Build history of the part. All positions in model axes, mm. Face numbers are marked on the shaded views. A direction names the side the tool comes from. Round coordinates to 2 decimals unless told otherwise and drop trailing zeros. Write each loop counter-clockwise with the first axis right and the second up, starting at its lowest first coordinate (ties: lowest second). Pieces come first, ordered by that corner, then holes. Notation, with made-up numbers: (10, -10) - (52, -10) arc R17 cw to (52, 6) - close; hole circle Ø2 at (-8.75, 44.5). An arc over 180 degrees is marked (long way). Answer as a JSON object with one key per item and string values. Group by question number.
Item 1: Slice it at C-C, the plane y = -14.5. List the corners of the cut face in (x, z), then the cut area to 3 significant figures.
Item 2: Slice it at A-A, the plane y = -4.5. List the corners of the cut face in (x, z).
Item 3: Which spindle directions (+Z, -Z, +X, -X, +Y, -Y) get a long thin tool onto all of the face, cutting with end or side? Do the marked faces 4 and 5. Say none if no direction does.
Item 4: Two-plate mould, pull along Z, no slides. Class the marked faces 1, 2 and 3: +Z half, -Z half, draft (parallel to the pull), parting line (faces both ways), or undercut.
Item 5: Slice it at B-B, the plane y = -10. List the corners of the cut face in (x, z), then the cut area to 3 significant figures.
Item 6: Flat gauge pins, fed straight in: pin 1 (6 mm diameter, centred on x = 13.5, y = -12, fed in from -Z); pin 2 (8 mm diameter, centred on x = 15, y = -11, fed in from -Z); pin 3 (4 mm diameter, centred on x = -0.5, y = -5.5, fed in from -Z). Where does each tip first touch, or does it go through?
Item 7: Probe line 1 (X direction, y = -11.5, z = 0); line 2 (X direction, y = -11.25, z = -2); line 3 (Z direction, x = 2.5, y = -7.75). List the from-to ranges inside material, lowest first. Write a range as from..to.
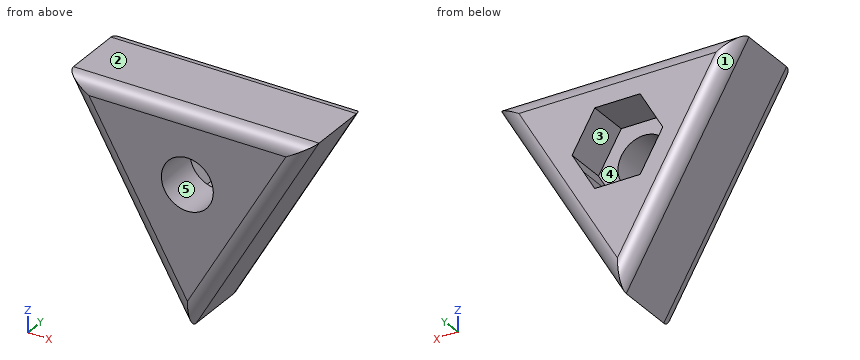
from build123d import *

# Parameters (mm, degrees)
F2_DEPTH = 15.875
F3_DEPTH = 7.62
F4_R     = 4.699
F5_DEPTH = 25.4
F6_R     = 2.54


with BuildPart() as f2:
    # F0 (on Front) → F2 (new body)
    with BuildSketch(Plane.XZ):
        Polygon((22.232984, 12.827), (-22.217016, 12.827), (0.007984, -25.667829), align=None)
    extrude(amount=F2_DEPTH)

    # F1 (on Front) → F3 (cut)
    with BuildSketch(Plane.XZ):
        Polygon((6.159173, -3.556), (8.21223, 0), (4.106115, 7.112), (-4.106115, 7.112), (-8.21223, 0), (-4.106115, -7.112), (4.106115, -7.112), align=None)
    extrude(amount=F3_DEPTH, mode=Mode.SUBTRACT)

    # F4 (on Front) → F5 (cut)
    with BuildSketch(Plane.XZ):
        Circle(F4_R)
    extrude(amount=F5_DEPTH, mode=Mode.SUBTRACT)

    # F6
    f6_edges = [f2.edges().sort_by_distance(p)[0] for p in [
        (-11.104516, 0, -6.420415),
        (0.007984, 0, 12.827),
        (11.120484, 0, -6.420415),
        (0.007984, -15.875, 12.827),
        (-11.104516, -15.875, -6.420415),
        (11.120484, -15.875, -6.420415),
    ]]
    fillet(f6_edges, radius=F6_R)


solid = f2.part
Geometry says:
{
 "1": {"outline": "(-21.73, 12.54) - (0.01, -25.1) - (21.74, 12.54) - close; hole circle Ø9.4 at (0, 0)", "area": "749 mm^2"},
 "2": {"outline": "(-22.22, 12.83) - (0.01, -25.67) - (22.23, 12.83) - close; hole (-8.21, 0) - (-4.11, -7.11) - (4.11, -7.11) - (6.16, -3.56) - (8.21, 0) - (4.11, 7.11) - (-4.11, 7.11) - close"},
 "3": {"face 4": "+Y", "face 5": "+Y, -Y"},
 "4": {"face 1": "-Z half", "face 2": "+Z half", "face 3": "undercut"},
 "5": {"outline": "(-22.22, 12.83) - (0.01, -25.67) - (22.23, 12.83) - close; hole circle Ø9.4 at (0, 0)", "area": "786 mm^2"},
 "6": {"pin 1": "stops at z = -7.5", "pin 2": "stops at z = -6.63", "pin 3": "stops at z = -25.67"},
 "7": {"line 1": "x = -14.81..-4.7, 4.7..14.83", "line 2": "x = -13.66..-4.25, 4.25..13.67", "line 3": "z = -21.35..-3.98, 3.98..12.83"}
}
